Verification items for the finished model (mm, model axes). Face numbers are marked on the shaded views. A direction names the side the tool comes from. Coordinates: 2 decimals unless noted, no trailing zeros. Loops run counter-clockwise (first coordinate to the right, second up) from the corner with the lowest first, then second, coordinate; pieces in that order, holes last.
Q1. Sectioned sample at D-D (y = 202). Enter the section's corners in (x, z) (3 decimals), then the cut area to 3 significant figures.
Q2. Material ranges on probe 1 along X at (y, z) = (166, 1) (3 decimals); probe 2 along X at (y, z) = (118.5, 11), recorded low to high.
Q3. Go/stop test with a flat-tipped pin: P1, Ø8, axis at x = -9.5, z = -3, coming from the +Y side. Record where the tip stops, or that it passes through.
Q4. Mould release check, pull along X, two halves, no side actions. Record for the marked faces 1, 2 and 3: +X half, -X half, draft (parallel to the pull), parting line (faces both ways), or undercut.
Q5. Sectioned sample at C-C (z = 0). Enter the section's corners in (x, y) (3 decimals), then the cut area to 3 significant figures.
Q6. Sectioned sample at B-B (y = 97). Enter the section's corners in (x, z) (3 decimals), then the cut area to 3 significant figures.
Q7. Access from +Z, -Z, +X, -X, +Y, -Y to the whole of each face (thin tool, end or side, straight path). Record for the marked faces 4 and 5.
Q8. Sectioned sample at A-A (x = 2.5). Enter the section's corners in (y, z) (3 decimals).
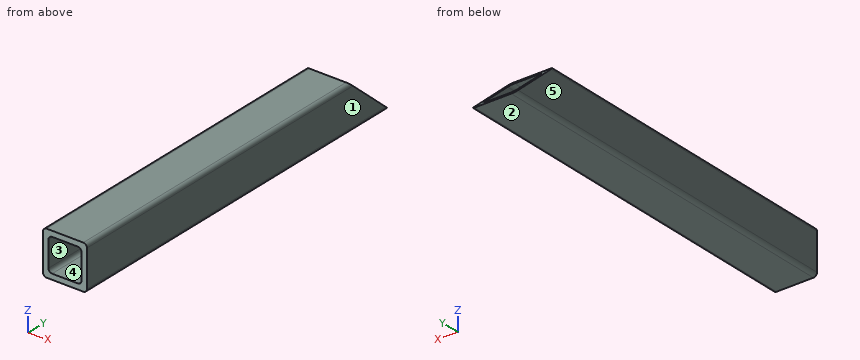
```python
from build123d import *

# Parameters (mm, degrees)
SKETCH1_W           = 25.4
SKETCH1_H           = 25.4
SKETCH1_W_2         = 19.05
SKETCH1_H_2         = 19.05
BOSS_EXTRUDE1_DEPTH = 1219.2
FILLET1_R           = 2.1082
SKETCH2_OUTSIDE_W   = 271.346
SKETCH2_OUTSIDE_H   = 1465.146
SKETCH2_OUTSIDE_W_2 = 161.404490431
SKETCH2_OUTSIDE_H_2 = 228.6
CUT_EXTRUDE1_DEPTH  = 1220.530684321
CUT_EXTRUDE2_DEPTH  = 231.35713577


with BuildPart() as part:
    # Sketch1 → Boss-Extrude1 (new body)
    with BuildSketch(Plane(origin=(0, 0, 0), x_dir=(1, 0, 0), z_dir=(0, 1, 0))):
        Rectangle(SKETCH1_W, SKETCH1_H)
        Rectangle(SKETCH1_W_2, SKETCH1_H_2, mode=Mode.SUBTRACT)
    extrude(amount=BOSS_EXTRUDE1_DEPTH)

    # Fillet1
    fillet1_edges = [part.edges().sort_by_distance(p)[0] for p in [
        (9.525, 609.6, 9.525),
        (9.525, 609.6, -9.525),
        (-9.525, 609.6, -9.525),
        (-9.525, 609.6, 9.525),
        (-12.7, 609.6, -12.7),
        (12.7, 609.6, -12.7),
        (12.7, 609.6, 12.7),
        (-12.7, 609.6, 12.7),
    ]]
    fillet(fillet1_edges, radius=FILLET1_R)

    # Sketch2 outside → Cut-Extrude1 (cut, through all)
    with BuildSketch(Plane(origin=(12.7, 0, 0), x_dir=(0, 0, -1), z_dir=(1, 0, 0))):
        with Locations((0, 609.6)):
            Rectangle(SKETCH2_OUTSIDE_W, SKETCH2_OUTSIDE_H)
        with Locations((42.327264621, 114.3)):
            Rectangle(SKETCH2_OUTSIDE_W_2, SKETCH2_OUTSIDE_H_2, mode=Mode.SUBTRACT)
    extrude(amount=-CUT_EXTRUDE1_DEPTH, mode=Mode.SUBTRACT)

    # Sketch3 → Cut-Extrude2 (cut, through all)
    with BuildSketch(Plane(origin=(12.7, 0, 0), x_dir=(0, 0, -1), z_dir=(1, 0, 0))):
        Polygon((-201.676, 0), (-14.872954341, 211.814744127), (-14.872954341, 228.6), (-0.069750097, 228.6), (15.452852017, 246.200976383), (26.360882017, 236.580998158), (10.838279903, 218.980021775), (-190.76797, -9.619978225), align=None)
    extrude(amount=-CUT_EXTRUDE2_DEPTH, mode=Mode.SUBTRACT)


solid = part.part
```
Geometry check:
1. outline: (-12.7, -10.592) arc R2.108 ccw to (-10.592, -12.7) - (10.592, -12.7) arc R2.108 ccw to (12.7, -10.592) - (12.7, 4.137) - (9.525, 4.137) - (9.525, -7.417) arc R2.108 cw to (7.417, -9.525) - (-7.417, -9.525) arc R2.108 cw to (-9.525, -7.417) - (-9.525, 4.137) - (-12.7, 4.137) - close
1. area: 167 mm2
2. probe 1: x = -12.7 to -9.525, 9.525 to 12.7
2. probe 2: x = -12.66 to 12.66
3. P1: stops at y = 214.63
4. face 1: +X half
4. face 2: draft
4. face 3: undercut
5. outline: (-12.7, 0) - (-9.525, 0) - (-9.525, 206.691) - (-12.7, 206.691) - close; (9.525, 0) - (12.7, 0) - (12.7, 206.691) - (9.525, 206.691) - close
5. area: 1,310 mm2
6. outline: (-12.7, -10.592) arc R2.108 ccw to (-10.592, -12.7) - (10.592, -12.7) arc R2.108 ccw to (12.7, -10.592) - (12.7, 10.592) arc R2.108 ccw to (10.592, 12.7) - (-10.592, 12.7) arc R2.108 ccw to (-12.7, 10.592) - close; hole (-9.525, -7.417) arc R2.108 ccw to (-7.417, -9.525) - (7.417, -9.525) arc R2.108 ccw to (9.525, -7.417) - (9.525, 7.417) arc R2.108 ccw to (7.417, 9.525) - (-7.417, 9.525) arc R2.108 ccw to (-9.525, 7.417) - close
6. area: 282 mm2
7. face 4: +Y, -Y
7. face 5: +Z, -Z, -X, +Y, -Y
8. outline: (0, -12.7) - (221.091, -12.7) - (217.491, -9.525) - (0, -9.525) - close; (0, 9.525) - (195.89, 9.525) - (192.29, 12.7) - (0, 12.7) - close
